from build123d import *

# Parameters (mm, degrees)
SKETCH1_W           = 240
SKETCH1_H           = 151
BOSS_EXTRUDE1_DEPTH = 5
SKETCH2_W           = 60
SKETCH2_H           = 40
CUT_EXTRUDE1_DEPTH  = 5
SKETCH4_R           = 2
CUT_EXTRUDE3_DEPTH  = 5
SKETCH5_R           = 4
SKETCH5_R_2         = 2
BOSS_EXTRUDE2_DEPTH = 5
CUT_EXTRUDE5_DEPTH  = 5
SKETCH12_R          = 2
CUT_EXTRUDE7_DEPTH  = 5
SKETCH13_R          = 2.5
CUT_EXTRUDE8_DEPTH  = 10
SKETCH16_W          = 5
SKETCH16_H          = 30
BOSS_EXTRUDE5_DEPTH = 5
CUT_EXTRUDE11_DEPTH = 5
SKETCH18_W          = 135.3
SKETCH18_H          = 20
CUT_EXTRUDE13_DEPTH = 10
SKETCH19_R          = 4
SKETCH19_R_2        = 2
BOSS_EXTRUDE6_DEPTH = 5
SKETCH20_W          = 24.8
SKETCH20_H          = 5
CUT_EXTRUDE14_DEPTH = 5
SKETCH21_W          = 25
SKETCH21_H          = 5
CUT_EXTRUDE15_DEPTH = 5
CUT_EXTRUDE16_DEPTH = 5
CUT_EXTRUDE17_DEPTH = 10


with BuildPart() as part:
    # Sketch1 → Boss-Extrude1 (new body)
    with BuildSketch(Plane.XY):
        Rectangle(SKETCH1_W, SKETCH1_H)
    extrude(amount=BOSS_EXTRUDE1_DEPTH)

    # Sketch2 → Cut-Extrude1 (cut)
    with BuildSketch(Plane(origin=(0, 0, 0), x_dir=(-1, 0, 0), z_dir=(0, 0, -1))):
        with Locations((12.301489704, 55.5)):
            Rectangle(SKETCH2_W, SKETCH2_H)
    extrude(amount=-CUT_EXTRUDE1_DEPTH, mode=Mode.SUBTRACT)

    # Sketch4 → Cut-Extrude3 (cut)
    with BuildSketch(Plane(origin=(0, 0, 0), x_dir=(-1, 0, 0), z_dir=(0, 0, -1))):
        with Locations((-107.8, 73)):
            Circle(SKETCH4_R)
        with Locations((-30.2, 73)):
            Circle(SKETCH4_R)
    extrude(amount=-CUT_EXTRUDE3_DEPTH, mode=Mode.SUBTRACT)

    # Sketch5 → Boss-Extrude2 (add)
    with BuildSketch(Plane(origin=(0, 0, 0), x_dir=(-1, 0, 0), z_dir=(0, 0, -1))):
        with Locations((-30.2, 73)):
            Circle(SKETCH5_R)
        with Locations((-30.2, 73)):
            Circle(SKETCH5_R_2, mode=Mode.SUBTRACT)
        with Locations((-107.8, 73)):
            Circle(SKETCH5_R)
        with Locations((-107.8, 73)):
            Circle(SKETCH5_R_2, mode=Mode.SUBTRACT)
    extrude(amount=-BOSS_EXTRUDE2_DEPTH)

    # Sketch8 → Cut-Extrude5 (cut)
    with BuildSketch(Plane(origin=(0, 0, 0), x_dir=(-1, 0, 0), z_dir=(0, 0, -1))):
        with BuildLine():
            Line((100, -60.5), (100, -40.5))
            ThreePointArc((100, -40.5), (105, -35.5), (110, -40.5))
            Line((110, -40.5), (110, -60.5))
            ThreePointArc((110, -60.5), (105, -65.5), (100, -60.5))
        make_face()
    extrude(amount=-CUT_EXTRUDE5_DEPTH, mode=Mode.SUBTRACT)

    # Sketch12 → Cut-Extrude7 (cut)
    with BuildSketch(Plane(origin=(0, 0, 0), x_dir=(-1, 0, 0), z_dir=(0, 0, -1))):
        with Locations((-28.16035742, -53.440416767)):
            Circle(SKETCH12_R)
    extrude(amount=-CUT_EXTRUDE7_DEPTH, mode=Mode.SUBTRACT)

    # Sketch13 → Cut-Extrude8 (cut)
    with BuildSketch(Plane(origin=(0, 0, 0), x_dir=(-1, 0, 0), z_dir=(0, 0, -1))):
        with Locations((110, -13)):
            Circle(SKETCH13_R)
    extrude(amount=-CUT_EXTRUDE8_DEPTH, mode=Mode.SUBTRACT)

    # Sketch16 → Boss-Extrude5 (add)
    with BuildSketch(Plane(origin=(0, 0, 0), x_dir=(-1, 0, 0), z_dir=(0, 0, -1))):
        with Locations((-122.5, 20.5)):
            Rectangle(SKETCH16_W, SKETCH16_H)
        with Locations((-122.5, -40.5)):
            Rectangle(SKETCH16_W, SKETCH16_H)
        with Locations((122.5, -40.5)):
            Rectangle(SKETCH16_W, SKETCH16_H)
        with Locations((122.5, 20.5)):
            Rectangle(SKETCH16_W, SKETCH16_H)
    extrude(amount=-BOSS_EXTRUDE5_DEPTH)

    # Sketch17 → Cut-Extrude11 (cut)
    with BuildSketch(Plane(origin=(0, 0, 0), x_dir=(-1, 0, 0), z_dir=(0, 0, -1))):
        Polygon((-120, 0.154989229), (-115, 0.154989229), (-115, 1.654989229), (-111.7, 1.654989229), (-111.7, 0.154989229), (-95, 0.154989229), (-95, -4.245010771), (-111.7, -4.245010771), (-111.7, -5.745010771), (-115, -5.745010771), (-115, -4.245010771), (-120, -4.245010771), align=None)
        Polygon((120, -4.245010771), (120, 0.154989229), (115, 0.154989229), (115, 1.654989229), (111.7, 1.654989229), (111.7, 0.154989229), (95, 0.154989229), (95, -4.245010771), (111.7, -4.245010771), (111.7, -5.745010771), (115, -5.745010771), (115, -4.245010771), align=None)
    extrude(amount=-CUT_EXTRUDE11_DEPTH, mode=Mode.SUBTRACT)

    # Sketch18 → Cut-Extrude13 (cut)
    with BuildSketch(Plane(origin=(0, 0, 0), x_dir=(-1, 0, 0), z_dir=(0, 0, -1))):
        with Locations((-9.8, -65.5)):
            Rectangle(SKETCH18_W, SKETCH18_H)
    extrude(amount=-CUT_EXTRUDE13_DEPTH, mode=Mode.SUBTRACT)

    # Sketch19 → Boss-Extrude6 (add)
    with BuildSketch(Plane(origin=(0, 0, 0), x_dir=(-1, 0, 0), z_dir=(0, 0, -1))):
        with Locations((-28.16035742, -53.440416767)):
            Circle(SKETCH19_R)
        with Locations((-28.16035742, -53.440416767)):
            Circle(SKETCH19_R_2, mode=Mode.SUBTRACT)
    extrude(amount=-BOSS_EXTRUDE6_DEPTH)

    # Sketch20 → Cut-Extrude14 (cut)
    with BuildSketch(Plane(origin=(0, 0, 0), x_dir=(-1, 0, 0), z_dir=(0, 0, -1))):
        with Locations((70.25, -73)):
            Rectangle(SKETCH20_W, SKETCH20_H)
    extrude(amount=-CUT_EXTRUDE14_DEPTH, mode=Mode.SUBTRACT)

    # Sketch21 → Cut-Extrude15 (cut)
    with BuildSketch(Plane(origin=(0, 0, 0), x_dir=(-1, 0, 0), z_dir=(0, 0, -1))):
        with Locations((-89.95, -73)):
            Rectangle(SKETCH21_W, SKETCH21_H)
    extrude(amount=-CUT_EXTRUDE15_DEPTH, mode=Mode.SUBTRACT)

    # Sketch22 → Cut-Extrude16 (cut)
    with BuildSketch(Plane(origin=(0, 0, 0), x_dir=(-1, 0, 0), z_dir=(0, 0, -1))):
        Polygon((68.25, -55.5), (68.25, -62.2), (66.75, -62.2), (66.75, -65.5), (68.25, -65.5), (68.25, -70.5), (72.65, -70.5), (72.65, -65.5), (74.15, -65.5), (74.15, -62.2), (72.65, -62.2), (72.65, -55.5), align=None)
        Polygon((-92.45, -55.5), (-92.45, -62.2), (-93.95, -62.2), (-93.95, -65.5), (-92.45, -65.5), (-92.45, -70.5), (-88.05, -70.5), (-88.05, -65.5), (-86.55, -65.5), (-86.55, -62.2), (-88.05, -62.2), (-88.05, -55.5), align=None)
    extrude(amount=-CUT_EXTRUDE16_DEPTH, mode=Mode.SUBTRACT)

    # Sketch23 → Cut-Extrude17 (cut)
    with BuildSketch(Plane(origin=(0, 0, 0), x_dir=(-1, 0, 0), z_dir=(0, 0, -1))):
        with BuildLine():
            Line((-100, 60.5), (-100, 40.5))
            ThreePointArc((-100, 40.5), (-107.5, 33), (-115, 40.5))
            Line((-115, 40.5), (-115, 60.5))
            ThreePointArc((-115, 60.5), (-107.5, 68), (-100, 60.5))
        make_face()
        with BuildLine():
            Line((100, 60.5), (100, 40.5))
            ThreePointArc((100, 40.5), (107.5, 33), (115, 40.5))
            Line((115, 40.5), (115, 60.5))
            ThreePointArc((115, 60.5), (107.5, 68), (100, 60.5))
        make_face()
    extrude(amount=-CUT_EXTRUDE17_DEPTH, mode=Mode.SUBTRACT)


solid = part.part
Geometry: final body of the model. Coordinates: model frame, mm. A direction names the side the tool comes from. Give positions to 0.01 mm unless a question says otherwise; leave off trailing zeros. Write each loop counter-clockwise with the first axis right and the second up, starting at its lowest first coordinate (ties: lowest second). Pieces come first, ordered by that corner, then holes.
(1) Cut plane A-A, the plane y = -13. Return loops of the section in (x, z), then the cut area to 4 significant figures.
(2) Mould query, pull axis Y, two halves, no side actions, for faces 1 (the flat face through (88.05, -68, 2)), 2 (the flat face through (-63, -70.5, 2)), 3 (the flat face through (-118, 0.155, 2)), 4 (the flat face through (115, 50, 2)). Classes: released by +Y, released by -Y, zero draft, split by the parting line, or undercut.
(3) Access query for faces 5 (the flat face through (123, 35.5, 2)), 6 (the flat face through (-122, -55.5, 2)), 7 (the flat face through (-68.25, -68, 2)), 8 (the flat face through (17.699, 55, 2)). Directions: +Z, -Z, +X, -X, +Y, -Y. A direction counts if a zero-diameter tool reaches every point of the face in a straight line with its end or side. Return the directions, or none.
(4) Cut plane D-D, the plane x = -77.5. Return loops of the section in (y, z), then the cut area to 3 significant figures.
(5) Cut plane C-C, the plane z = 1.65. Give the number of separate pieces and of enclosed holes in the cut face, then the cut area to 3 significant figures.
(6) Cut plane B-B, the plane x = -102.5. Return loops of the section in (y, z).
(7) First-contact query: P1, Ø2.5, axis at y = -62, z = 2, coming from the +X side; P2, Ø1, axis at x = -6, y = 13.5, coming from the -Z side; P3, Ø1.5, axis at y = -57.5, z = 2.5, coming from the -X side; P4, Ø1.6, axis at x = 93, z = 3, coming from the +Y side. Flat tips, straight axial feed; report the tip coordinate or a pass-through.
(8) Ray query, line 1 (X direction, y = 0.5, z = 2.6); line 2 (Y direction, x = 107.8, z = 3.2); line 3 (X direction, y = 61, z = 2.6). Return the intervals inside material, ascending.
Values follow:
1. outline: (-120, 0) - (-112.5, 0) - (-112.5, 5) - (-120, 5) - close; (-107.5, 0) - (120, 0) - (120, 5) - (-107.5, 5) - close
1. area: 1,175 mm2
2. face 1: zero draft
2. face 2: released by -Y
2. face 3: undercut
2. face 4: undercut
3. face 5: +Z, -Z, +X, +Y
3. face 6: +Z, -Z, -X, -Y
3. face 7: +Z, -Z, -Y
3. face 8: +Z, -Z, +Y
4. outline: (-70.5, 0) - (75.5, 0) - (75.5, 5) - (-70.5, 5) - close
4. area: 730 mm2
5. separate pieces: 1
5. enclosed holes: 7
5. area: 29,800 mm2
6. outline: (-75.5, 0) - (-64.83, 0) - (-64.83, 5) - (-75.5, 5) - close; (-36.17, 0) - (-4.25, 0) - (-4.25, 5) - (-36.17, 5) - close; (0.15, 0) - (34.91, 0) - (34.91, 5) - (0.15, 5) - close; (66.09, 0) - (75.5, 0) - (75.5, 5) - (66.09, 5) - close
7. P1: stops at x = 120
7. P2: stops at z = 0
7. P3: stops at x = -120
7. P4: stops at y = 75.5
8. line 1: x = -120 to -115, -111.7 to 111.7, 115 to 120
8. line 2: y = -75.5 to -4.25, 0.15 to 33.01, 67.99 to 71, 75 to 77
8. line 3: x = -120 to -114.98, -100.02 to -42.3, 17.7 to 100.02, 114.98 to 120
